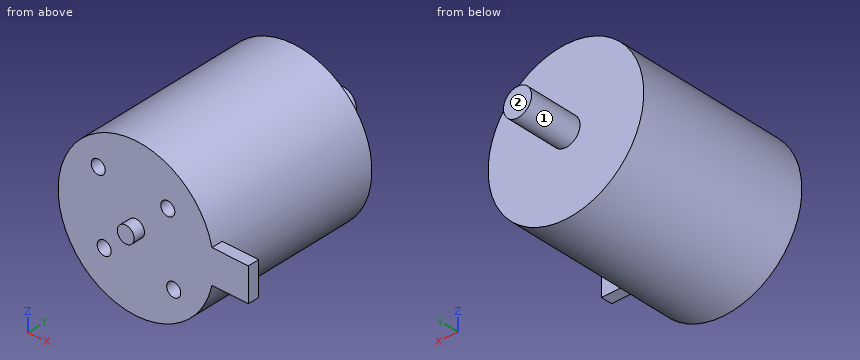
```python
from build123d import *

# Parameters (mm, degrees)
SKETCH_3_R          = 1.25
CUT_EXTRUDE_1_DEPTH = 5
EXTRUDE_1_DEPTH     = 2


with BuildPart() as part:
    # Эскиз2 → Повернуть1 (revolve)
    with BuildSketch(Plane(origin=(0, 0, 0), x_dir=(0, 0, -1), z_dir=(1, 0, 0))):
        Polygon((0, 0), (0, 31), (0, 40.5), (2.5, 40.5), (2.5, 31), (13.85, 31), (13.85, 0), (1.5, 0), (1.5, -2), (0, -2), align=None)
    revolve(axis=Axis((0, 0, 0), (0, 1, 0)))

    # Эскиз3 → Вырез-Вытянуть1 (cut)
    with BuildSketch(Plane.XZ):
        with Locations(Location((5.65685425, 5.65685425, 0), (0, 0, 270))):
            Circle(SKETCH_3_R)
        with Locations(Location((6.717514421, -6.717514421, 0), (0, 0, 270))):
            Circle(SKETCH_3_R)
        with Locations(Location((-6.717514421, 6.717514421, 0), (0, 0, 90))):
            Circle(SKETCH_3_R)
        with Locations(Location((-5.65685425, -5.65685425, 0), (0, 0, 90))):
            Circle(SKETCH_3_R)
    extrude(amount=-CUT_EXTRUDE_1_DEPTH, mode=Mode.SUBTRACT)

    # Эскиз4 → Бобышка-Вытянуть1 (add)
    with BuildSketch(Plane.XZ):
        with BuildLine():
            Line((13.521187078, -3), (13.85, -3))
            Line((13.85, -3), (20, -3))
            Line((20, -3), (20, 3))
            Line((20, 3), (13.521187078, 3))
            ThreePointArc((13.521187078, 3), (13.767551362, 1.50898293), (13.85, 0))
            ThreePointArc((13.85, 0), (13.767551362, -1.50898293), (13.521187078, -3))
        make_face()
    extrude(amount=-EXTRUDE_1_DEPTH)


solid = part.part
```
Can you work these out from the model? Positions are in its coordinate system, mm. Face numbers are marked on the shaded views. A direction names the side the tool comes from. Coordinates: 2 decimals unless noted, no trailing zeros. Loops run counter-clockwise (first coordinate to the right, second up) from the corner with the lowest first, then second, coordinate; pieces in that order, holes last. Notation, with made-up numbers: (7, 17) -> (20, 17) arc R18 cw to (20, 50) -> close; hole circle Ø8 at (20, -25.5). An arc over 180 degrees is marked (long way). Answer as a JSON object with one key per item and string values.
1) Imagine slicing it at C-C (y = 33.5). Please give me the cut outline in (x, z), then the cut area to 3 significant figures.
Results:
{"outline": "circle Ø5 at (0, 0)", "area": "19.6 mm^2"}
2) For P1, Ø8, axis at y = 7, z = 6, coming from the -X side; P2, Ø1.2, axis at x = 6.5, z = -7, coming from the -Y side; P3, Ø4, axis at x = 6.72, z = -6.72, coming from the -Y side, each with a flat end and sliding along its axis, tell me the tip position at first contact or that it passes through.
Results:
{"P1": "stops at x = -13.7", "P2": "stops at y = 5", "P3": "stops at y = 0"}
3) If I drill on line 1 (Y direction, x = -8, z = -9.75); line 2 (Z direction, x = -12, y = 24.5); line 3 (Y direction, x = 15.5, z = 2), over which ranges is the centre line in solid material (lowest first)?
Results:
{"line 1": "y = 0 to 31", "line 2": "z = -6.92 to 6.92", "line 3": "y = 0 to 2"}
4) Imagine slicing it at B-B (z = 0). Please give me the cut outline in (x, y).
Results:
{"outline": "(-13.85, 0) -> (-1.5, 0) -> (-1.5, -2) -> (1.5, -2) -> (1.5, 0) -> (20, 0) -> (20, 2) -> (13.85, 2) -> (13.85, 31) -> (2.5, 31) -> (2.5, 40.5) -> (-2.5, 40.5) -> (-2.5, 31) -> (-13.85, 31) -> close"}
5) Imagine slicing it at D-D (y = 9). Please give me the cut outline in (x, z).
Results:
{"outline": "circle Ø27.7 at (0, 0)"}
6) For the marked faces 1 and 2, which set-ups out of +Z, -Z, +X, -X, +Y, -Y let a thin tool reach every point of the face, with its end or its side?
Results:
{"face 1": "+Y", "face 2": "+Z, -Z, +X, -X, +Y"}
7) Imagine slicing it at A-A (x = 0). Please give me the cut outline in (y, z).
Results:
{"outline": "(-2, -1.5) -> (0, -1.5) -> (0, -13.85) -> (31, -13.85) -> (31, -2.5) -> (40.5, -2.5) -> (40.5, 2.5) -> (31, 2.5) -> (31, 13.85) -> (0, 13.85) -> (0, 1.5) -> (-2, 1.5) -> close"}
